Autodesk Inventor part; units mm, degrees
ref_plane "YZ Plane" through (0, 0, 0) normal (1, 0, 0) x (0, 1, 0)
ref_plane "XZ Plane" through (0, 0, 0) normal (0, 1, 0) x (-1, 0, 0)
ref_plane "XY Plane" through (0, 0, 0) normal (0, 0, 1) x (1, 0, 0)
sketch "Sketch1" plane through (0, 0, 0) normal (0, 0, 1) x (1, 0, 0)
  circle A0 centre (0, 0) radius 3.9624
  dimension "d0" = 7.9248
extrude "Extrusion1" add sketch "Sketch1" along normal blind 4.826
sketch "Sketch2" plane through (0, 0, 0) normal (0, 0, -1) x (-1, 0, 0)
  circle A0 centre (0, 0) radius 3.9624
  circle A1 centre (0, 0) radius 2.413
  dimension "d3" = 4.826
extrude "Extrusion2" add sketch "Sketch2" along normal blind 41.275 contours A1
sketch "Sketch3" plane through (0, 0, 4.826) normal (0, 0, 1) x (1, 0, 0)
  circle A0 centre (0, 0) radius 3.9624
  line L0 (-1.1457, 1.9844) -> (1.1457, 1.9844)
  line L1 (1.1457, 1.9844) -> (2.2914, 0)
  line L2 (2.2914, 0) -> (1.1457, -1.9844)
  line L3 (1.1457, -1.9844) -> (-1.1457, -1.9844)
  line L4 (-1.1457, -1.9844) -> (-2.2914, 0)
  line L5 (-2.2914, 0) -> (-1.1457, 1.9844)
  dimension "d6" = 3.9688
extrude "Extrusion3" cut sketch "Sketch3" against normal blind 3.175 contours L0 L1 L2 L3 L4 L5
thread "Thread1"
chamfer "Chamfer1" distance 0.508 angle 45 1 edges at (2.413, 0, -41.275)
chamfer "Chamfer2" distance 0.508 angle 45 1 edges at (-3.9624, 0, 4.826)
properties part number "10-32 x1625" material "Steel"
Geometry check sheet. Reference: the model listing, model coordinates, mm. A direction names the side the tool comes from. Round coordinates to 2 decimals unless told otherwise and drop trailing zeros. Loops run counter-clockwise (first coordinate to the right, second up) from the corner with the lowest first, then second, coordinate; pieces in that order, holes last. Notation, with made-up numbers: (66.5, 89) - (74.5, 89) arc R27 cw to (74.5, 116) - close; hole circle Ø3 at (-13.75, 49). An arc over 180 degrees is marked (long way). Write item = value, one per line. Start each with the question number.
1. Section check B-B on z = -2.5. Enter the section's corners in (x, y), then the cut area to 3 significant figures.
2. Depth check by flat-ended pin: pin 1 (0.7 mm diameter, centred on x = -0.5, z = 3, fed in from -Y); pin 2 (4 mm diameter, centred on x = 3, z = -15.5, fed in from -Y); pin 3 (1.5 mm diameter, centred on x = 1.5, z = -29.5, fed in from +Y). Enter the tip coordinate at first touch or a pass-through.
3. Thickness scan on line 1 (Z direction, x = 0.75, y = 2.75); line 2 (Z direction, x = 0.25, y = 0.25) (3 decimals); line 3 (Y direction, x = 0.75, z = -17). Record the ranges inside material, lowest first.
4. Set-up check for faces 1 (the face through (1.71, 1.01, 3.26)), 2 (the face through (0, 0, -41.275)), 3 (the face through (2, 2, 0)): record each of +Z, -Z, +X, -X, +Y, -Y from which the full face is reachable in a straight line by a thin tool's end or side.
5. Mould release check, pull along X, two halves, no side actions. Record for faces 4 (the face through (-1.71, -1.01, 3.26)), 5 (the face through (1.915, 1.468, -20.098)), 6 (the face through (-2, -1, 4.826)): released by +X, released by -X, zero draft, split by the parting line, or undercut.
6. Section check A-A on x = 0. Enter the section's corners in (y, z) (3 decimals).
Working result:
q1.outline = circle Ø4.83 at (0, 0)
q1.area = 18.3 mm^2
q2.pin_1 = -3.96
q2.pin_2 = -2.2
q2.pin_3 = 2.29
q3.line_1 = 0 to 4.83
q3.line_2 = -41.275 to 1.651
q3.line_3 = -2.29 to 2.29
q4.face_1 = +Z
q4.face_2 = -Z, +X, -X, +Y, -Y
q4.face_3 = -Z
q5.face_4 = undercut
q5.face_5 = split by the parting line
q5.face_6 = zero draft
q6.outline = (-3.962, 0) - (-2.413, 0) - (-2.413, -40.767) - (-1.905, -41.275) - (1.905, -41.275) - (2.413, -40.767) - (2.413, 0) - (3.962, 0) - (3.962, 4.318) - (3.454, 4.826) - (1.984, 4.826) - (1.984, 1.651) - (-1.984, 1.651) - (-1.984, 4.826) - (-3.454, 4.826) - (-3.962, 4.318) - close
